The model under review builds one solid part; all positions refer to its coordinate system, in mm. A direction names the side the tool comes from. Round coordinates to 2 decimals unless told otherwise and drop trailing zeros. Loops run counter-clockwise (first coordinate to the right, second up) from the corner with the lowest first, then second, coordinate; pieces in that order, holes last. Notation, with made-up numbers: (9, 42) -> (32, 42) arc R17 ccw to (32, 54) -> close; hole circle Ø11 at (-11, 27.25). An arc over 180 degrees is marked (long way). Use CSV: the item, a comma, the result in double quotes. Start each with the question number.
```python
from build123d import *

# Parameters (mm, degrees)
CROQUIS1_R              = 1.5
SALIENTE_EXTRUIR1_DEPTH = 2


with BuildPart() as part:
    # Croquis1 → Saliente-Extruir1 (new body)
    with BuildSketch(Plane.XY):
        with BuildLine():
            Line((-806.293781222, 387.093592203), (-805.087201617, 388.694777419))
            ThreePointArc((-805.087201617, 388.694777419), (-803.111242937, 389.859794234), (-800.889769824, 389.288187645))
            Line((-800.889769824, 389.288187645), (-789.110634699, 380.442131133))
            ThreePointArc((-789.110634699, 380.442131133), (-787.230269134, 379.189584745), (-785.220630898, 378.157111371))
            Line((-785.220630898, 378.157111371), (-761.350873045, 367.552403578))
            ThreePointArc((-761.350873045, 367.552403578), (-758.375650619, 367.099552447), (-755.400428194, 367.552403578))
            Line((-755.400428194, 367.552403578), (-731.530670341, 378.157111371))
            ThreePointArc((-731.530670341, 378.157111371), (-729.521032104, 379.189584745), (-727.640666539, 380.442131133))
            Line((-727.640666539, 380.442131133), (-715.861531414, 389.288187645))
            ThreePointArc((-715.861531414, 389.288187645), (-713.640058301, 389.859794234), (-711.664099621, 388.694777419))
            Line((-711.664099621, 388.694777419), (-710.457520016, 387.093592203))
            Line((-710.457520016, 387.093592203), (-709.250181935, 385.491400454))
            ThreePointArc((-709.250181935, 385.491400454), (-708.674856636, 383.271490166), (-709.835721429, 381.293765761))
            Line((-709.835721429, 381.293765761), (-722.491711895, 371.715934755))
            ThreePointArc((-722.491711895, 371.715934755), (-723.477203121, 370.919812191), (-724.410312611, 370.062892842))
            Line((-724.410312611, 370.062892842), (-732.976662667, 361.68062014))
            ThreePointArc((-732.976662667, 361.68062014), (-737.407061656, 350.984690814), (-732.976662667, 340.288761488))
            Line((-732.976662667, 340.288761488), (-724.410312611, 331.906488787))
            ThreePointArc((-724.410312611, 331.906488787), (-723.477203121, 331.049569437), (-722.491711895, 330.253446873))
            Line((-722.491711895, 330.253446873), (-709.835721429, 320.675615867))
            ThreePointArc((-709.835721429, 320.675615867), (-708.674856636, 318.697891463), (-709.250181935, 316.477981174))
            Line((-709.250181935, 316.477981174), (-710.457520016, 314.875789425))
            Line((-710.457520016, 314.875789425), (-711.664099621, 313.274604209))
            ThreePointArc((-711.664099621, 313.274604209), (-713.640058301, 312.109587395), (-715.861531414, 312.681193984))
            Line((-715.861531414, 312.681193984), (-727.640666539, 321.527250495))
            ThreePointArc((-727.640666539, 321.527250495), (-729.521032104, 322.779796883), (-731.530670341, 323.812270257))
            Line((-731.530670341, 323.812270257), (-755.400428194, 334.41697805))
            ThreePointArc((-755.400428194, 334.41697805), (-758.375650619, 334.869829182), (-761.350873045, 334.41697805))
            Line((-761.350873045, 334.41697805), (-785.220630898, 323.812270257))
            ThreePointArc((-785.220630898, 323.812270257), (-787.230269134, 322.779796883), (-789.110634699, 321.527250495))
            Line((-789.110634699, 321.527250495), (-800.889769824, 312.681193984))
            ThreePointArc((-800.889769824, 312.681193984), (-803.111242937, 312.109587395), (-805.087201617, 313.274604209))
            Line((-805.087201617, 313.274604209), (-806.293781222, 314.875789425))
            Line((-806.293781222, 314.875789425), (-807.501119304, 316.477981174))
            ThreePointArc((-807.501119304, 316.477981174), (-808.076444603, 318.697891463), (-806.915579809, 320.675615867))
            Line((-806.915579809, 320.675615867), (-794.259589343, 330.253446873))
            ThreePointArc((-794.259589343, 330.253446873), (-793.274098117, 331.049569437), (-792.340988627, 331.906488787))
            Line((-792.340988627, 331.906488787), (-783.774638572, 340.288761488))
            ThreePointArc((-783.774638572, 340.288761488), (-779.344239583, 350.984690814), (-783.774638572, 361.68062014))
            Line((-783.774638572, 361.68062014), (-792.340988627, 370.062892842))
            ThreePointArc((-792.340988627, 370.062892842), (-793.274098117, 370.919812191), (-794.259589343, 371.715934755))
            Line((-794.259589343, 371.715934755), (-806.915579809, 381.293765761))
            ThreePointArc((-806.915579809, 381.293765761), (-808.076444603, 383.271490166), (-807.501119304, 385.491400454))
            Line((-807.501119304, 385.491400454), (-806.293781222, 387.093592203))
        make_face()
        with Locations((-802.300603672, 384.084517088)):
            Circle(CROQUIS1_R, mode=Mode.SUBTRACT)
        with Locations((-783.935934024, 370.245745896)):
            Circle(CROQUIS1_R, mode=Mode.SUBTRACT)
        with Locations((-766.36200572, 357.002841046)):
            Circle(CROQUIS1_R, mode=Mode.SUBTRACT)
        with Locations((-773.625650619, 366.234690814)):
            Circle(CROQUIS1_R, mode=Mode.SUBTRACT)
        with Locations(Location((-750.389295519, 357.002841046, 0), (0, 0, 180))):
            Circle(CROQUIS1_R, mode=Mode.SUBTRACT)
        with Locations(Location((-743.125650619, 366.234690814, 0), (0, 0, 180))):
            Circle(CROQUIS1_R, mode=Mode.SUBTRACT)
        with Locations(Location((-732.815367214, 370.245745896, 0), (0, 0, 180))):
            Circle(CROQUIS1_R, mode=Mode.SUBTRACT)
        with Locations(Location((-714.450697566, 384.084517088, 0), (0, 0, 180))):
            Circle(CROQUIS1_R, mode=Mode.SUBTRACT)
        with Locations((-714.450697566, 317.884864541)):
            Circle(CROQUIS1_R, mode=Mode.SUBTRACT)
        with Locations((-732.815367214, 331.723635733)):
            Circle(CROQUIS1_R, mode=Mode.SUBTRACT)
        with Locations((-743.125650619, 335.734690814)):
            Circle(CROQUIS1_R, mode=Mode.SUBTRACT)
        with Locations((-750.389295519, 344.966540583)):
            Circle(CROQUIS1_R, mode=Mode.SUBTRACT)
        with Locations(Location((-766.36200572, 344.966540583, 0), (0, 0, 180))):
            Circle(CROQUIS1_R, mode=Mode.SUBTRACT)
        with Locations(Location((-773.625650619, 335.734690814, 0), (0, 0, 180))):
            Circle(CROQUIS1_R, mode=Mode.SUBTRACT)
        with Locations(Location((-783.935934024, 331.723635733, 0), (0, 0, 180))):
            Circle(CROQUIS1_R, mode=Mode.SUBTRACT)
        with Locations(Location((-802.300603672, 317.884864541, 0), (0, 0, 180))):
            Circle(CROQUIS1_R, mode=Mode.SUBTRACT)
    extrude(amount=SALIENTE_EXTRUIR1_DEPTH)


solid = part.part
```
1. The part is to be moulded in two halves that separate along X. For faces 5 (the face through (-723.49, 331.06, 0.99)), 6 (the face through (-762, 351, 2)), 7 (the face through (-773.12, 329.19, 0.99)), say which applies: pulls with the +X half, pulls with the -X half, needs draft (parallel to the pull), parting line crosses it, or undercut.
2. Take a section at C-C, the plane x = -781. Give the boundary of the cut face in (y, z).
3. Take a section at B-B, the plane z = 0.4. Count the separate pieces of the cut face and the enclosed holes in it, then the cut area to 3 significant figures.
4. For line 1 along X through (y, z) = (370, 0.25); line 2 along X through (y, z) = (356.5, 1.1); line 3 along X through (y, z) = (356, 1.45), list the stretches that pass through material, from the lowest coordinate up. Write a range as from..to.
5. Clearance check with a flat-ended pin moving along its axis: P1, Ø3.5, axis at x = -714.45, y = 384.08, coming from the -Z side. State where the tip first meets the part, or that it passes through.
6. Take a section at A-A, the plane x = -729. Give the boundary of the cut face in (y, z).
7. For faces 1 (the face through (-800.5, 376.44, 0.99)), 2 (the face through (-803.079, 312.105, 0.986)), 3 (the face through (-773.453, 372.929, 0.986)), 4 (the face through (-723.5, 370.9, 1)), list the 3-axis set-ups (+Z, -Z, +X, -X, +Y, -Y) from which the entire face can be reached by the end or side of a thin tool; tool diameter is ignored.
Results:
1,face 5,"pulls with the +X half"
1,face 6,"needs draft"
1,face 7,"undercut"
2,outline,"(325.69, 0) -> (344.1, 0) -> (344.1, 2) -> (325.69, 2) -> close; (357.87, 0) -> (376.28, 0) -> (376.28, 2) -> (357.87, 2) -> close"
3,separate pieces,"1"
3,enclosed holes,"16"
3,area,"3,050 mm²"
4,line 1,"-792.28..-785.42, -782.46..-766.86, -749.89..-734.3, -731.34..-724.47"
4,line 2,"-780.39..-767.78, -764.95..-751.8, -748.98..-736.37"
4,line 3,"-780.2..-767.48, -765.25..-751.5, -749.27..-736.55"
5,P1,"z = 0"
6,outline,"(322.46, 0) -> (336.4, 0) -> (336.4, 2) -> (322.46, 2) -> close; (365.57, 0) -> (379.51, 0) -> (379.51, 2) -> (365.57, 2) -> close"
7,face 1,"+Z, -Z, -X"
7,face 2,"+Z, -Z, -Y"
7,face 3,"+Z, -Z, +Y"
7,face 4,"+Z, -Z, +X"
